from build123d import *

# Parameters (mm, degrees)
F1_DEPTH = 18


# Not quite as in the source:
# - ends of sketch curves that miss each other by under 0.0002 mm in the source are joined


with BuildPart() as f1:
    # F0 (on Front) → F1 (new body)
    with BuildSketch(Plane.XZ):
        with BuildLine():
            Line((195.0137715405, 361), (195.0137715405, 379))
            Line((195.0137715405, 379), (169.0137715405, 379))
            Line((169.0137715405, 379), (169.0137715405, 361.0021361967))
            Line((169.0137715405, 361.0021361967), (169.0137715405, 361))
            ThreePointArc((169.0137715405, 361), (165.0116353441, 357.0021367671), (161.0137721109, 361.0042723931))
            Line((161.0137721109, 361.0042723931), (-161.0000017113, 361.1762435819))
            ThreePointArc((-161.0000017113, 361.1762435819), (-165.0021373372, 357.1783803487), (-169.0000005704, 361.1805159746))
            Line((-169.0000005704, 361.1805159746), (-169.0000005704, 379.1805159746))
            Line((-169.0000005704, 379.1805159746), (-195.0000005704, 379.1805159746))
            Line((-195.0000005704, 379.1805159746), (-195.0000005704, 361.1805160001))
            ThreePointArc((-195.0000005704, 361.1805160001), (-199, 357.1805165706), (-202.9999994296, 361.1805160001))
            Line((-202.9999994296, 361.1805160001), (-215.9862284595, 361.1805160001))
            Line((-215.9862284595, 361.1805160001), (-215.9862284595, -0.2833213137))
            ThreePointArc((-215.9862284595, -0.2833213137), (-211.9862284595, -4.2833213137), (-215.9862284595, -8.2833213137))
            Line((-215.9862284595, -8.2833213137), (-233.9862284595, -8.2833213137))
            ThreePointArc((-233.9862284595, -8.2833213137), (-237.9862284595, -4.2833213137), (-233.9862284595, -0.2833213137))
            Line((-233.9862284595, -0.2833213137), (-233.9862284595, 361.1805160001))
            Line((-233.9862284595, 361.1805160001), (-244.90749278, 361.1805160001))
            Line((-244.90749278, 361.1805160001), (-274.9862284595, 331.0746893941))
            Line((-274.9862284595, 331.0746893941), (-254.9862284595, -376.2833213137))
            Line((-254.9862284595, -376.2833213137), (-233.9862284595, -376.2833213137))
            Line((-233.9862284595, -376.2833213137), (-215.9862284595, -376.2833213137))
            Line((-215.9862284595, -376.2833213137), (-194.9862284595, -376.2833213137))
            Line((-194.9862284595, -376.2833213137), (-174.9862284595, 210.3365797868))
            Line((-174.9862284595, 210.3365797868), (-134.9862284595, 250.3365797868))
            Line((-134.9862284595, 250.3365797868), (135, 250.3365797868))
            Line((135, 250.3365797868), (175, 210.3365797868))
            Line((175, 210.3365797868), (195, -376.2833213137))
            Line((195, -376.2833213137), (216.0083907756, -375.6897371419))
            Line((216.0083907756, -375.6897371419), (234.0083907756, -375.6897371419))
            Line((234.0083907756, -375.6897371419), (255, -376.2833213137))
            Line((255, -376.2833213137), (275, 331))
            Line((275, 331), (245, 361))
            Line((245, 361), (234.0083907756, 361))
            Line((234.0083907756, 361), (234.0083907756, 0.3102628581))
            ThreePointArc((234.0083907756, 0.3102628581), (238.0083907756, -3.6897371419), (234.0083907756, -7.6897371419))
            Line((234.0083907756, -7.6897371419), (216.0083907756, -7.6897371419))
            ThreePointArc((216.0083907756, -7.6897371419), (212.0083907756, -3.6897371419), (216.0083907756, 0.3102628581))
            Line((216.0083907756, 0.3102628581), (216.0083907756, 361))
            Line((216.0083907756, 361), (203.0137715405, 361))
            ThreePointArc((203.0137715405, 361), (199.0137715405, 357), (195.0137715405, 361))
        make_face()
    extrude(amount=F1_DEPTH)


solid = f1.part
Geometry: final body of the model. Coordinates: model frame, mm. A direction names the side the tool comes from. Give positions to 0.01 mm unless a question says otherwise; leave off trailing zeros. Write each loop counter-clockwise with the first axis right and the second up, starting at its lowest first coordinate (ties: lowest second). Pieces come first, ordered by that corner, then holes.
(1) Cut plane B-B, the plane z = -158. Return loops of the section in (x, y), then the cut area to 3 significant figures.
(2) Ray query, line 1 (X direction, y = -3.75, z = 96); line 2 (X direction, y = -5.5, z = 104); line 3 (X direction, y = -14.25, z = 281). Return the intervals inside material, ascending.
(3) Cut plane C-C, the plane x = -225. Return loops of the section in (y, z).
(4) Mould query, pull axis X, two halves, no side actions, for faces 1 (the flat face through (182, -9, 379)), 2 (the flat face through (-155.266, -8.874, 230.057)), 3 (the flat face through (-2, -9, 250.337)), 4 (the flat face through (-259.736, -8.874, 346.338)). Classes: released by +X, released by -X, zero draft, split by the parting line, or undercut.
(5) First-contact query: P1, Ø9, axis at y = -6.5, z = 172.5, coming from the -X side; P2, Ø3, axis at y = -16, z = 66, coming from the -X side; P3, Ø10, axis at y = -8.5, z = 135, coming from the +X side. Flat tips, straight axial feed; report the tip coordinate or a pass-through.
(6) Cut plane D-D, the plane x = -26.5. Return loops of the section in (y, z).
(7) Cut plane A-A, the plane z = 95.5. Return loops of the section in (x, y), then the cut area to 3 significant figures.
(8) Access query for faces 5 (the flat face through (154.72, -8.874, 230.617)), 6 (the flat face through (195.014, -9, 370)), 7 (the flat face through (216.008, -9, 178)). Directions: +Z, -Z, +X, -X, +Y, -Y. A direction counts if a zero-diameter tool reaches every point of the face in a straight line with its end or side. Return the directions, or none.
Values follow:
1. outline: (-261.16, -18) - (-187.54, -18) - (-187.54, 0) - (-261.16, 0) - close; (187.56, -18) - (261.17, -18) - (261.17, 0) - (187.56, 0) - close
1. area: 2,650 mm2
2. line 1: x = -268.34 to -233.99, -215.99 to -178.88, 178.9 to 216.01, 234.01 to 268.35
2. line 2: x = -268.57 to -233.99, -215.99 to -178.61, 178.63 to 216.01, 234.01 to 268.58
2. line 3: x = -273.57 to -233.99, -215.99 to 216.01, 234.01 to 273.59
3. outline: (-18, -376.28) - (0, -376.28) - (0, -8.28) - (-18, -8.28) - close
4. face 1: zero draft
4. face 2: undercut
4. face 3: undercut
4. face 4: released by -X
5. P1: stops at x = -270.63
5. P2: stops at x = -267.53
5. P3: stops at x = 269.6
6. outline: (-18, 250.34) - (0, 250.34) - (0, 361.1) - (-18, 361.1) - close
7. outline: (-268.33, -18) - (-233.99, -18) - (-233.99, 0) - (-268.33, 0) - close; (-215.99, -18) - (-178.9, -18) - (-178.9, 0) - (-215.99, 0) - close; (178.92, -18) - (216.01, -18) - (216.01, 0) - (178.92, 0) - close; (234.01, -18) - (268.34, -18) - (268.34, 0) - (234.01, 0) - close
7. area: 2,570 mm2
8. face 5: -Z, +Y, -Y
8. face 6: +Z, +X, +Y, -Y
8. face 7: +Z, +Y, -Y
